Geometry: final body of the model. Coordinates: model frame, mm. Face numbers are marked on the shaded views. A direction names the side the tool comes from. Give positions to 0.01 mm unless a question says otherwise; leave off trailing zeros. Write each loop counter-clockwise with the first axis right and the second up, starting at its lowest first coordinate (ties: lowest second). Pieces come first, ordered by that corner, then holes.
Q1. Cut plane A-A on y = 9. Count the separate pieces of the cut face and the enclosed holes in it, plus the area to 3 significant figures.
Q2. Pin query (flat end, axial travel): pin 1 (6 mm diameter, centred on x = 9.5, y = 11.5, fed in from +Z). Return the tip coordinate at first contact, or that it passes through.
Q3. Line query: L1, parallel to Y at x = 14, z = 1.25; L2, parallel to X at y = 13, z = 3.5. Output: solid intervals per line, ascending.
Q4. Draft query along X for the marked faces 1, 2 and 3. Return one class per face: pulls with the +X half, pulls with the -X half, needs draft (parallel to the pull), parting line crosses it, or undercut.
Q5. Cut plane C-C on x = 14. Return the cut outline in (y, z).
Q6. Cut plane B-B on z = 14. Return the cut outline in (x, y).
Q7. Reachability of the marked faces 4 and 5 from +Z, -Z, +X, -X, +Y, -Y: full face, straight path, thin tool, end or side. Return the list, or none.
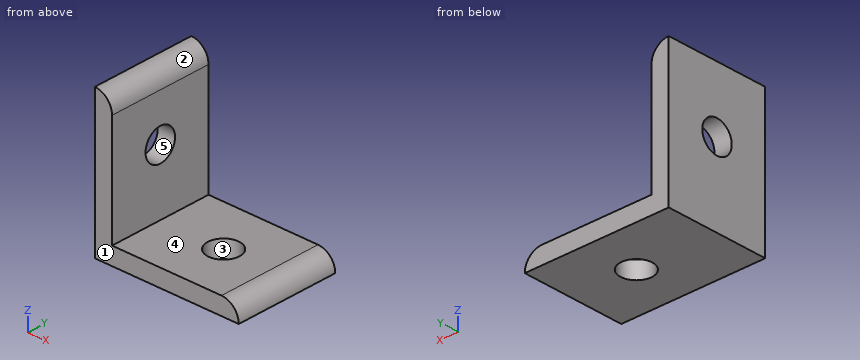
```python
from build123d import *

# Parameters (mm, degrees)
BOSS_EXTRUDE1_DEPTH = 18
SKETCH3_R           = 2.75
CUT_EXTRUDE2_DEPTH  = 38.854986461
FILLET1_R           = 3


with BuildPart() as part:
    # Sketch2 → Boss-Extrude1 (new body)
    with BuildSketch(Plane(origin=(0, 0, 0), x_dir=(-1, 0, 0), z_dir=(0, 1, 0))):
        Polygon((0, 0), (0, 25), (-3, 25), (-3, 3), (-25, 3), (-25, 0), align=None)
    extrude(amount=BOSS_EXTRUDE1_DEPTH)

    # Sketch3 → Cut-Extrude2 (cut, through all)
    with BuildSketch(Plane.XY.offset(3)):
        with Locations((14, 9)):
            Circle(SKETCH3_R)
    cut_extrude2 = extrude(amount=-CUT_EXTRUDE2_DEPTH, mode=Mode.SUBTRACT)

    # Mirror1: Cut-Extrude2 across plane
    add(cut_extrude2.mirror(Plane(origin=(0, 0, 0), x_dir=(0.7071067811865465, 0, 0.7071067811865486), z_dir=(-0.7071067811865488, 0, 0.7071067811865464))), mode=Mode.SUBTRACT)

    # Fillet1
    fillet1_edges = [part.edges().sort_by_distance(p)[0] for p in [
        (3, 9, 25),
        (25, 9, 3),
    ]]
    fillet(fillet1_edges, radius=FILLET1_R - 0.0001)  # a hair under: the kernel refuses the full size


solid = part.part
```
Data:
1. separate pieces: 3
1. enclosed holes: 0
1. area: 104 mm2
2. pin 1: stops at z = 3
3. L1: y = 0 to 6.25, 11.75 to 18
3. L2: x = 0 to 3
4. face 1: needs draft
4. face 2: pulls with the +X half
4. face 3: undercut
5. outline: (0, 0) - (6.25, 0) - (6.25, 3) - (0, 3) - close; (11.75, 0) - (18, 0) - (18, 3) - (11.75, 3) - close
6. outline: (0, 0) - (3, 0) - (3, 6.25) - (0, 6.25) - close; (0, 11.75) - (3, 11.75) - (3, 18) - (0, 18) - close
7. face 4: +Z, +X, +Y, -Y
7. face 5: +X, -X
